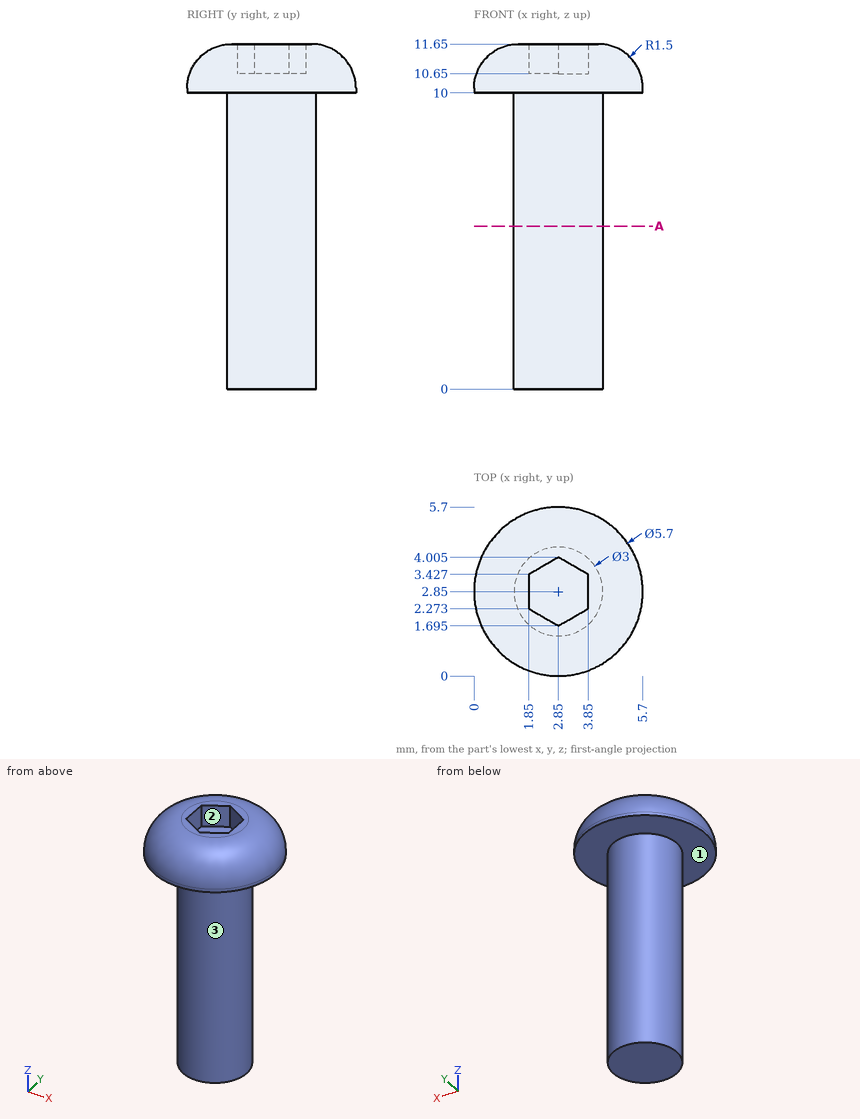
Drawing for the job (mm, zero at the part's lowest x, y, z). Give positions to 0.01 mm unless a question says otherwise; leave off trailing zeros. Order: outer loops, then holes, each group sorted by start corner. A loop starts at its lowest first (then second) coordinate and runs counter-clockwise, first axis right, second up. Notation, with made-up numbers: M 2.5,74.5 L 46.5,74.5 A18 cw 46.5,104.5 Z; hole C 37,88 d5. An arc over 180 degrees is marked long. Use a Markdown table: item, result. Add a question column.
(1) Mould opens along X. For the marked faces 1, 2 and 3 say: +X half, -X half, draft (parallel to the pull), parting line (faces both ways), or undercut.
(2) Saw through at A-A, the plane z = 5.5. Give the cut face in (x, y).
(3) Probe line 1 along Z through (x, y) = (2.45, 3.35); line 2 along Z through (x, y) = (0.6, 2.25) (1 decimal); line 3 along Y through (x, z) = (1.95, 3). List the from-to ranges inside material, lowest first. Write a range as [from, to].
(4) Drop flat-ended pins along their axis: P1, Ø0.5, axis at y = 3, z = 11.5, coming from the -X side (1 decimal); P2, Ø0.5, axis at y = 3, z = 11, coming from the +X side; P3, Ø1.5, axis at x = 3, z = 5, coming from the -Y side. Give the stop position or say it passes through.
Answer key:
| question | item | result |
|---|---|---|
| 1 | face 1 | draft |
| 1 | face 2 | undercut |
| 1 | face 3 | parting line |
| 2 | outline | C 2.85,2.85 d3 |
| 3 | line 1 | [0, 10.65] |
| 3 | line 2 | [10, 11.3] |
| 3 | line 3 | [1.65, 4.05] |
| 4 | P1 | x = 0.5 |
| 4 | P2 | x = 5.57 |
| 4 | P3 | y = 1.35 |
